Source: three-view drawing plus pictorial views. Frame: mm from the lowest corner of the part. Round coordinates to 2 decimals unless told otherwise and drop trailing zeros. Loops run counter-clockwise (first coordinate to the right, second up) from the corner with the lowest first, then second, coordinate; pieces in that order, holes last. Notation, with made-up numbers: (8.5, -29.75) -> (15.5, -29.75) arc R15 cw to (15.5, -10.75) -> close; hole circle Ø7 at (82.25, 28). An arc over 180 degrees is marked (long way). Answer in a Markdown table with one row per item.
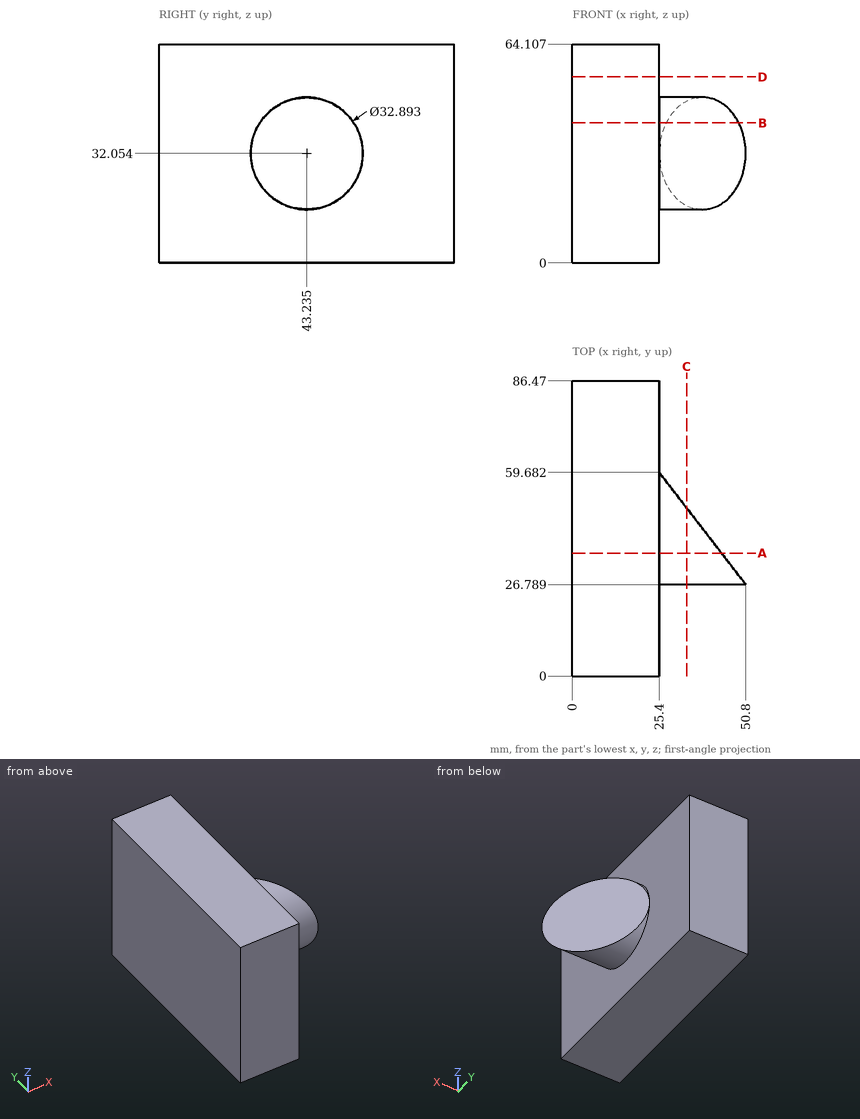
Item 1: Cut plane B-B (z = 41). Output: boundary loops of the cut face in (x, y) (1 decimal), then the cut area to 3 significant figures.
Answer:
| item | result |
|---|---|
| outline | (0, 0) -> (25.4, 0) -> (25.4, 29.4) -> (48.8, 29.4) -> (27.4, 57) -> (25.4, 57) -> (25.4, 86.5) -> (0, 86.5) -> close |
| area | 2,550 mm² |
Item 2: Cut plane A-A (y = 36). Output: boundary loops of the cut face in (x, z), then the cut area to 3 significant figures.
Answer:
| item | result |
|---|---|
| outline | (0, 0) -> (25.4, 0) -> (25.4, 17.28) -> (43.69, 17.28) -> (43.69, 46.82) -> (25.4, 46.82) -> (25.4, 64.11) -> (0, 64.11) -> close |
| area | 2,170 mm² |
Item 3: Cut plane C-C (x = 33.5). Output: boundary loops of the cut face in (y, z) (1 decimal).
Answer:
| item | result |
|---|---|
| outline | (49.2, 16.7) -> (49.2, 47.4) arc R16.4 ccw (long way) to start |
Item 4: Pin query (flat end, axial travel): pin 1 Ø1.5 at (y, z) = (57, 38) entering from +X; pin 2 Ø1.5 at (x, z) = (27, 46.5) entering from +Y; pin 3 Ø12 at (y, z) = (67, 24.5) entering from +X. Return the tip coordinate at first contact, or that it passes through.
Answer:
| item | result |
|---|---|
| pin 1 | stops at x = 28.05 |
| pin 2 | stops at y = 52.34 |
| pin 3 | stops at x = 25.4 |
Item 5: Cut plane D-D (z = 54.5). Output: boundary loops of the cut face in (x, y), then the cut area to 3 significant figures.
Answer:
| item | result |
|---|---|
| outline | (0, 0) -> (25.4, 0) -> (25.4, 86.47) -> (0, 86.47) -> close |
| area | 2,200 mm² |
Item 6: Line query: probe 1 along X at (y, z) = (75, 61); probe 2 along Y at (x, z) = (31.5, 40.5) (1 decimal); probe 3 along Z at (x, y) = (45, 31) (1 decimal). Output: solid intervals per line, ascending. Write a range as [from, to].
Answer:
| item | result |
|---|---|
| probe 1 | x = [0, 25.4] |
| probe 2 | y = [29.1, 51.8] |
| probe 3 | z = [21.1, 43] |
